Print and shaded views of the part. All mm, measured from the part's lowest x, y and z. Round coordinates to 2 decimals unless told otherwise and drop trailing zeros. Order: outer loops, then holes, each group sorted by start corner. A loop starts at its lowest first (then second) coordinate and runs counter-clockwise, first axis right, second up. Notation, with made-up numbers: (11, 7.25) - (68, 7.25) arc R18 ccw to (68, 26.25) - close; hole circle Ø5 at (11, -26.75). An arc over 180 degrees is marked (long way). Return JSON: item names as keys, results as strings. Group by question number.
Item 1: Saw through at A-A on x = 414. List the corners of the cut face in (y, z), and give its area (3 significant figures).
Item 2: Drop flat-ended pins along their axis: pin 1 (1.5 mm diameter, centred on x = 249.5, z = 15.5, fed in from +Y); pin 2 (2 mm diameter, centred on y = 105, z = 13.5, fed in from -X); pin 3 (5 mm diameter, centred on y = 387, z = 15, fed in from +X). Give the stop position or say it passes through.
Item 3: Saw through at C-C on z = 12.5. List the corners of the cut face in (x, y), and give its area (3 significant figures).
Item 4: Probe probe 1 along Y at (x, z) = (357, 14). List the from-to ranges inside material, lowest first.
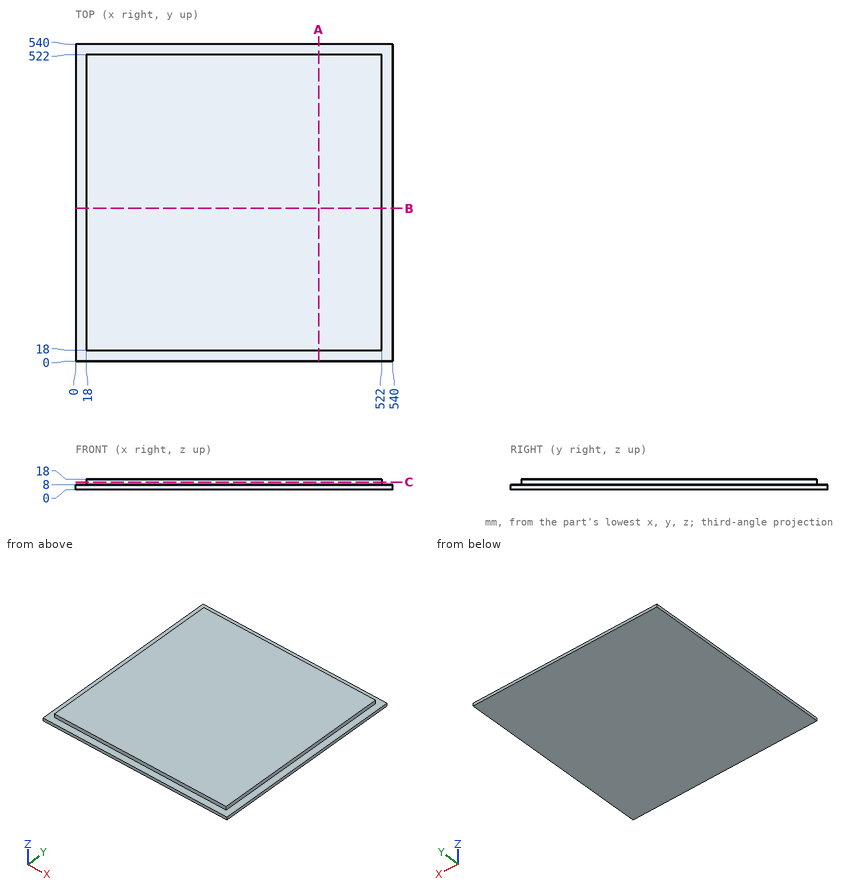
Filled in:
{
 "1": {"outline": "(0, 0) - (540, 0) - (540, 8) - (522, 8) - (522, 18) - (18, 18) - (18, 8) - (0, 8) - close", "area": "9,360 mm^2"},
 "2": {"pin 1": "stops at y = 522", "pin 2": "stops at x = 18", "pin 3": "stops at x = 522"},
 "3": {"outline": "(18, 18) - (522, 18) - (522, 522) - (18, 522) - close", "area": "254,000 mm^2"},
 "4": {"probe 1": "y = 18 to 522"}
}
